```python
from build123d import *

# Parameters (mm, degrees)
SKETCH1_W           = 240
SKETCH1_H           = 158
BOSS_EXTRUDE1_DEPTH = 5
CUT_EXTRUDE1_DEPTH  = 6


with BuildPart() as part:
    # Sketch1 → Boss-Extrude1 (new body)
    with BuildSketch(Plane(origin=(0, 0, 0), x_dir=(1, 0, 0), z_dir=(0, 1, 0))):
        with Locations((0, -79)):
            Rectangle(SKETCH1_W, SKETCH1_H)
    extrude(amount=BOSS_EXTRUDE1_DEPTH)

    # Sketch5 → Cut-Extrude1 (cut, through all)
    with BuildSketch(Plane.XZ):
        with BuildLine():
            Line((120, 158), (120, 128))
            ThreePointArc((120, 128), (98.786796564, 136.786796564), (90, 158))
            Line((90, 158), (120, 158))
        make_face()
    extrude(amount=-CUT_EXTRUDE1_DEPTH, mode=Mode.SUBTRACT)


solid = part.part
```
Geometry check sheet. Reference: the model listing, model coordinates, mm. Round coordinates to 2 decimals unless told otherwise and drop trailing zeros. Order: outer loops, then holes, each group sorted by start corner. A loop starts at its lowest first (then second) coordinate and runs counter-clockwise, first axis right, second up. Notation, with made-up numbers: (31.25, 47) - (70.25, 47) arc R20 cw to (70.25, 70) - close; hole circle Ø6 at (81.5, -27.75). An arc over 180 degrees is marked (long way). Use a Markdown table: item, result. Add a question column.
(1) Depth check by flat-ended pin: pin 1 (1 mm diameter, centred on x = -92, y = 3, fed in from -Z). Enter the tip coordinate at first touch or a pass-through.
(2) Sectioned sample at A-A, the plane y = 2.5. Enter the section's corners in (x, z).
(3) Material ranges on line 1 along X through (y, z) = (0.85, 148); line 2 along Z through (x, y) = (107, 1.05); line 3 along Z through (x, y) = (94.5, 2.7), recorded low to high. Write a range as [from, to].
(4) Sectioned sample at B-B, the plane z = 130.5. Enter the section's corners in (x, y).
Answers below:
| question | item | result |
|---|---|---|
| 1 | pin 1 | z = 0 |
| 2 | outline | (-120, 0) - (120, 0) - (120, 128) arc R30 cw to (90, 158) - (-120, 158) - close |
| 3 | line 1 | [-120, 91.72] |
| 3 | line 2 | [0, 130.96] |
| 3 | line 3 | [0, 142.2] |
| 4 | outline | (-120, 0) - (108.01, 0) - (108.01, 5) - (-120, 5) - close |
